from build123d import *

# Parameters (mm, degrees)
F0_W     = 20
F0_H     = 4
F1_DEPTH = 2
F2_W     = 4
F2_H     = 4
F3_DEPTH = 4


with BuildPart() as f1:
    # F0 (on Front) → F1 (new body)
    with BuildSketch(Plane.XZ):
        Rectangle(F0_W, F0_H)
    extrude(amount=F1_DEPTH)

    # F2 (on face) → F3 (join)
    with BuildSketch(Plane.XZ.offset(2)):
        with Locations((-8, 0)):
            Rectangle(F2_W, F2_H)
        with Locations((8, 0)):
            Rectangle(F2_W, F2_H)
    extrude(amount=F3_DEPTH)


solid = f1.part
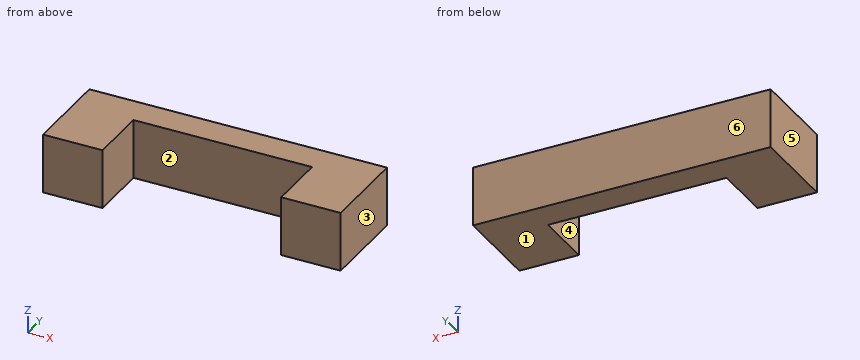
CAD build for the part. Positions are in the model's coordinates, mm. Face numbers are marked on the shaded views. A direction names the side the tool comes from. Round coordinates to 2 decimals unless told otherwise and drop trailing zeros. Loops run counter-clockwise (first coordinate to the right, second up) from the corner with the lowest first, then second, coordinate; pieces in that order, holes last.
(1) Cut at B-B (z = -1.3). Give the cut face in (x, y), plus the area to 3 significant figures.
(2) Drop a flat-ended pin along its axis: pin 1 (2 mm diameter, centred on x = 2.5, z = 1, fed in from -Y). Give the stop position or say it passes through.
(3) Two-plate mould, pull along X, no slides. Class the marked faces 3, 4, 5 and 6: +X half, -X half, draft (parallel to the pull), parting line (faces both ways), or undercut.
(4) Wall check: line 1 along X through (y, z) = (-3.9, -1.7); line 2 along Y through (x, z) = (-3.75, 1.45). Give the ranges that are in metal, low to high.
(5) Which spindle directions (+Z, -Z, +X, -X, +Y, -Y) get a long thin tool onto all of the face, cutting with end or side? Do the marked faces 1 and 2. Say none if no direction does.
(6) Cut at A-A (y = -3.45). Give the cut face in (x, z).
(7) Cut at C-C (x = -3.25). Give the cut face in (y, z).
Findings below:
1. outline: (-10, -6) - (-6, -6) - (-6, -2) - (6, -2) - (6, -6) - (10, -6) - (10, 0) - (-10, 0) - close
1. area: 72.0 mm2
2. pin 1: stops at y = -2
3. face 3: +X half
3. face 4: undercut
3. face 5: -X half
3. face 6: draft
4. line 1: x = -10 to -6, 6 to 10
4. line 2: y = -2 to 0
5. face 1: -Z, +X, -X, +Y, -Y
5. face 2: +Z, -Z, -Y
6. outline: (-10, -2) - (-6, -2) - (-6, 2) - (-10, 2) - close; (6, -2) - (10, -2) - (10, 2) - (6, 2) - close
7. outline: (-2, -2) - (0, -2) - (0, 2) - (-2, 2) - close
